Read the model definition and answer for the solid it produces. Units are mm, in the model's axes. A direction names the side the tool comes from. Coordinates: 2 decimals unless noted, no trailing zeros. Order: outer loops, then holes, each group sorted by start corner. A loop starts at its lowest first (then second) coordinate and runs counter-clockwise, first axis right, second up. Notation, with made-up numbers: (4.25, -23.5) -> (57.25, -23.5) arc R13 ccw to (57.25, -17.5) -> close; hole circle Ø6 at (-28.75, -0.5). An arc over 180 degrees is marked (long way). Use CSV: the item, a comma, the result in double quotes.
```python
from build123d import *

# Parameters (mm, degrees)
SKETCH_1_W      = 15
SKETCH_1_H      = 13.566666666
EXTRUDE_1_DEPTH = 1.6
EXTRUDE_2_DEPTH = 2.5


with BuildPart() as part:
    # 草图1 → 凸台-拉伸1 (new body)
    with BuildSketch(Plane(origin=(0, 0, 0), x_dir=(1, 0, 0), z_dir=(0, 1, 0))):
        Rectangle(SKETCH_1_W, SKETCH_1_H)
    extrude(amount=EXTRUDE_1_DEPTH)

    # 草图2 → 凸台-拉伸2 (add)
    with BuildSketch(Plane(origin=(0, 1.6, 0), x_dir=(1, 0, 0), z_dir=(0, 1, 0))):
        Polygon((-8.3, -4), (-8.3, 4), (-2.5, 3.75), (-2.5, -3.75), align=None)
    extrude(amount=EXTRUDE_2_DEPTH)


solid = part.part
```
Item 1: Straight lines are drawn through the part: line 1 along Y through (x, z) = (1, -1.75); line 2 along X through (y, z) = (1.8, -3.25); line 3 along X through (y, z) = (0.7, 0). For each, find the intervals that lie inside material, in ascending order.
Return value:
line 1,"y = 0 to 1.6"
line 2,"x = -8.3 to -2.5"
line 3,"x = -7.5 to 7.5"
Item 2: Find section D-D, the plane x = 4. Give the vertices of the cut face in (y, z), then the cut area to 3 significant figures.
Return value:
outline,"(0, -6.78) -> (1.6, -6.78) -> (1.6, 6.78) -> (0, 6.78) -> close"
area,"21.7 mm^2"
Item 3: Find section A-A, the plane z = -3.25. Give the vertices of the cut face in (x, y).
Return value:
outline,"(-8.3, 1.6) -> (-7.5, 1.6) -> (-7.5, 0) -> (7.5, 0) -> (7.5, 1.6) -> (-2.5, 1.6) -> (-2.5, 4.1) -> (-8.3, 4.1) -> close"
Item 4: A tool of negligible diameter and unlimited length cuts with its end or side. For faces 1 (the flat face through (-2.5, 3, 0)), 2 (the flat face through (-7.5, 1, 0)), 3 (the flat face through (-5.359, 2.832, 3.873)), 4 (the flat face through (-5.441, 2.832, -3.877)), from which of +Z, -Z, +X, -X, +Y, -Y can it reach the whole face along a straight path? Write none if from no direction.
Return value:
face 1,"+Z, -Z, +X, +Y"
face 2,"+Z, -Z, -X, -Y"
face 3,"+Z, +X, +Y"
face 4,"-Z, +X, +Y"
Item 5: Find section B-B, the plane x = -4. Give the vertices of the cut face in (y, z), then the cut area to 3 significant figures.
Return value:
outline,"(0, -6.78) -> (1.6, -6.78) -> (1.6, -3.81) -> (4.1, -3.81) -> (4.1, 3.81) -> (1.6, 3.81) -> (1.6, 6.78) -> (0, 6.78) -> close"
area,"40.8 mm^2"
Item 6: Each of these flat-tipped pins is pushed along its axis until it touches: P1, Ø4, axis at x = 1.5, z = 3, coming from the +Y side; P2, Ø0.5, axis at y = 1, z = -1, coming from the -X side. Where does it stop, or does it pass through?
Return value:
P1,"stops at y = 1.6"
P2,"stops at x = -7.5"
Item 7: Find section C-C, the plane y = 1.3. Give the vertices of the cut face in (x, z).
Return value:
outline,"(-7.5, -6.78) -> (7.5, -6.78) -> (7.5, 6.78) -> (-7.5, 6.78) -> close"
